Source: CAD feature listing. Evaluate the final solid. Frame: model axes, mm. A direction names the side the tool comes from. Round coordinates to 2 decimals unless told otherwise and drop trailing zeros. Loops run counter-clockwise (first coordinate to the right, second up) from the corner with the lowest first, then second, coordinate; pieces in that order, holes last.
Item 1: Section query B-B on z = 46.99. Return loops of the section in (x, y), then the cut area to 3 significant figures.
Item 2: Access query for faces 5 (the cylindrical face through (13.91, 0.8, -30.83)), 6 (the flat face through (0.783, 25.561, 17.647)), 7 (the cylindrical face through (1.36, 1.43, -3.94)). Directions: +Z, -Z, +X, -X, +Y, -Y. A direction counts if a zero-diameter tool reaches every point of the face in a straight line with its end or side. Return the directions, or none.
Item 3: Section query A-A on y = 12.7. Return loops of the section in (x, z), then the cut area to 3 significant figures.
Item 4: Ray query, L1, parallel to Y at x = 1, z = 14.5; L2, parallel to Y at x = 4.5, z = -15; L3, parallel to X at y = 97.5, z = 24. Return the intervals inside material, ascending.
Item 5: Section query D-D on x = 14. Return loops of the section in (y, z), then the cut area to 3 significant figures.
Item 6: Pull-direction query (Z, two-part tool) for faces 1 (the flat face through (20, 1.588, -4)), 2 (the flat face through (1, 61, -40.64)), 3 (the cylindrical face through (0.78, 105.47, 17.82)), 4 (the flat face through (0.783, 46.246, 17.647)); classes: released by +Z, released by -Z, zero draft, split by the parting line, or undercut.
Item 7: First-contact query: P1, Ø1.7, axis at x = 0.5, y = 102, coming from the +Z side; P2, Ø1.5, axis at x = 15, z = -25, coming from the +Y side; P3, Ø2, axis at x = 3, z = 13.5, coming from the +Y side. Flat tips, straight axial feed; report the tip coordinate or a pass-through.
```python
from build123d import *

# Parameters (mm, degrees)
SKETCH2_R                     = 14.2875
SKETCH2_R_2                   = 2.54
BOSS_EXTRUDE1_DEPTH           = 1.5875
SKETCH7_W                     = 1.5875
SKETCH7_H                     = 27.94
CUT_EXTRUDE1_DEPTH            = 0.00254
EDGE_FLANGE2_STRIP_W          = 12.7
EDGE_FLANGE2_STRIP_H          = 1.5875
EDGE_FLANGE2_STRIP_CUT_DEPTH  = 72.39
EDGE_FLANGE2_RELIEF_W         = 13.49375
EDGE_FLANGE2_RELIEF_H         = 0.79375
EDGE_FLANGE2_RELIEF_CUT_DEPTH = 1.5875
EDGE_FLANGE2_DEPTH            = 72.39
SKETCH14_R                    = 2.54
CUT_EXTRUDE2_DEPTH            = 2.54


# Sheet-metal steps are written as plain solids
with BuildPart() as part:
    # Sketch2 → Boss-Extrude1 (new body)
    with BuildSketch(Plane(origin=(0, 0, 0), x_dir=(0, 0, -1), z_dir=(1, 0, 0))):
        Polygon((-59.69, 95.25), (-59.69, 0), (40.64, 0), (40.64, 95.25), (40.64, 120.65), (-31.75, 120.65), (-31.75, 95.25), align=None)
        with Locations((0, 80.264)):
            Circle(SKETCH2_R, mode=Mode.SUBTRACT)
        with Locations((-46.99, 80.264)):
            Circle(SKETCH2_R_2, mode=Mode.SUBTRACT)
        with Locations((-46.99, 63.373)):
            Circle(SKETCH2_R_2, mode=Mode.SUBTRACT)
        with Locations((-17.272, 107.95)):
            Circle(SKETCH2_R_2, mode=Mode.SUBTRACT)
        with Locations((-2.794, 107.95)):
            Circle(SKETCH2_R_2, mode=Mode.SUBTRACT)
        with Locations((11.684, 107.95)):
            Circle(SKETCH2_R_2, mode=Mode.SUBTRACT)
        with Locations((26.162, 107.95)):
            Circle(SKETCH2_R_2, mode=Mode.SUBTRACT)
        with Locations((-46.99, 46.482)):
            Circle(SKETCH2_R_2, mode=Mode.SUBTRACT)
        with Locations((-46.99, 29.591)):
            Circle(SKETCH2_R_2, mode=Mode.SUBTRACT)
        with Locations((-46.99, 12.7)):
            Circle(SKETCH2_R_2, mode=Mode.SUBTRACT)
        with BuildLine():
            Line((-27.305, 64.866068321), (-8.255, 53.867545693))
            ThreePointArc((-8.255, 53.867545693), (-7.62, 52.76769343), (-8.255, 51.667841167))
            Line((-8.255, 51.667841167), (-27.305, 40.669318539))
            ThreePointArc((-27.305, 40.669318539), (-28.575, 40.669318539), (-29.21, 41.769170802))
            Line((-29.21, 41.769170802), (-29.21, 63.766216058))
            ThreePointArc((-29.21, 63.766216058), (-28.575, 64.866068321), (-27.305, 64.866068321))
        make_face(mode=Mode.SUBTRACT)
        with BuildLine():
            Line((-6.35, 43.235640486), (-6.35, 21.238595229))
            ThreePointArc((-6.35, 21.238595229), (-6.985, 20.138742967), (-8.255, 20.138742967))
            Line((-8.255, 20.138742967), (-27.305, 31.137265595))
            ThreePointArc((-27.305, 31.137265595), (-27.94, 32.237117857), (-27.305, 33.33697012))
            Line((-27.305, 33.33697012), (-8.255, 44.335492748))
            ThreePointArc((-8.255, 44.335492748), (-6.985, 44.335492748), (-6.35, 43.235640486))
        make_face(mode=Mode.SUBTRACT)
        with BuildLine():
            Line((8.255, 20.138742967), (27.305, 31.137265595))
            ThreePointArc((27.305, 31.137265595), (27.94, 32.237117857), (27.305, 33.33697012))
            Line((27.305, 33.33697012), (8.255, 44.335492748))
            ThreePointArc((8.255, 44.335492748), (6.985, 44.335492748), (6.35, 43.235640486))
            Line((6.35, 43.235640486), (6.35, 21.238595229))
            ThreePointArc((6.35, 21.238595229), (6.985, 20.138742967), (8.255, 20.138742967))
        make_face(mode=Mode.SUBTRACT)
        with BuildLine():
            Line((8.255, 51.667841167), (27.305, 40.669318539))
            ThreePointArc((27.305, 40.669318539), (28.575, 40.669318539), (29.21, 41.769170802))
            Line((29.21, 41.769170802), (29.21, 63.766216058))
            ThreePointArc((29.21, 63.766216058), (28.575, 64.866068321), (27.305, 64.866068321))
            Line((27.305, 64.866068321), (8.255, 53.867545693))
            ThreePointArc((8.255, 53.867545693), (7.62, 52.76769343), (8.255, 51.667841167))
        make_face(mode=Mode.SUBTRACT)
    extrude(amount=BOSS_EXTRUDE1_DEPTH)

    # Sketch7 → Cut-Extrude1 (cut)
    with BuildSketch(Plane(origin=(0, 0, 0), x_dir=(-1, 0, 0), z_dir=(0, -1, 0))):
        with Locations((-0.79375, -45.72)):
            Rectangle(SKETCH7_W, SKETCH7_H)
    extrude(amount=-CUT_EXTRUDE1_DEPTH, mode=Mode.SUBTRACT)

    # Edge-Flange2 strip (across the edge) → Edge-Flange2 strip cut (cut)
    with BuildSketch(Plane(origin=(1.5875, 0, 31.75), x_dir=(0, 1, 0), z_dir=(0, 0, -1))):
        with Locations((-1.5875, -0.79375)):
            Rectangle(EDGE_FLANGE2_STRIP_W, EDGE_FLANGE2_STRIP_H)
    extrude(amount=EDGE_FLANGE2_STRIP_CUT_DEPTH, mode=Mode.SUBTRACT)

    # Edge-Flange2 relief (on the sheet) → Edge-Flange2 relief cut (cut)
    with BuildSketch(Plane(origin=(1.5875, 4.7625, 31.75), x_dir=(0, 1, 0), z_dir=(1, 0, 0))):
        with Locations((-5.953125, 0.396875)):
            Rectangle(EDGE_FLANGE2_RELIEF_W, EDGE_FLANGE2_RELIEF_H)
    extrude(amount=-EDGE_FLANGE2_RELIEF_CUT_DEPTH, mode=Mode.SUBTRACT)

    # Edge-Flange2 section (across the edge) → Edge-Flange2 (add)
    with BuildSketch(Plane(origin=(1.5875, 0, 31.75), x_dir=(0, 1, 0), z_dir=(0, 0, -1))):
        with BuildLine():
            Line((0, 3.175), (0, 23.8125))
            Line((0, 23.8125), (1.5875, 23.8125))
            Line((1.5875, 23.8125), (1.5875, 3.175))
            ThreePointArc((1.5875, 3.175), (2.51743597, 0.92993597), (4.7625, 0))
            Line((4.7625, 0), (4.7625, -1.5875))
            ThreePointArc((4.7625, -1.5875), (1.394903955, -0.192596045), (0, 3.175))
        make_face()
    extrude(amount=EDGE_FLANGE2_DEPTH)

    # Sketch14 → Cut-Extrude2 (cut)
    with BuildSketch(Plane(origin=(0, 1.5875, 0), x_dir=(1, 0, 0), z_dir=(0, 1, 0))):
        with Locations(Location((15.08125, -19.685, 0), (0, 0, 180))):
            Circle(SKETCH14_R)
        with Locations(Location((15.08125, -7.62, 0), (0, 0, 180))):
            Circle(SKETCH14_R)
        with Locations(Location((15.08125, 4.445, 0), (0, 0, 180))):
            Circle(SKETCH14_R)
        with Locations(Location((15.08125, 16.51, 0), (0, 0, 180))):
            Circle(SKETCH14_R)
        with Locations(Location((15.08125, 28.575, 0), (0, 0, 180))):
            Circle(SKETCH14_R)
    extrude(amount=-CUT_EXTRUDE2_DEPTH, mode=Mode.SUBTRACT)


solid = part.part
```
Data:
1. outline: (0, 0) - (1.59, 0) - (1.59, 10.16) - (0, 10.16) - close; (0, 15.24) - (1.59, 15.24) - (1.59, 27.05) - (0, 27.05) - close; (0, 32.13) - (1.59, 32.13) - (1.59, 43.94) - (0, 43.94) - close; (0, 49.02) - (1.59, 49.02) - (1.59, 60.83) - (0, 60.83) - close; (0, 65.91) - (1.59, 65.91) - (1.59, 77.72) - (0, 77.72) - close; (0, 82.8) - (1.59, 82.8) - (1.59, 95.25) - (0, 95.25) - close
1. area: 111 mm2
2. face 5: +Y, -Y
2. face 6: +X, -X
2. face 7: -Z, -X, -Y
3. outline: (0, -40.64) - (1.59, -40.64) - (1.59, 44.45) - (0, 44.45) - close; (0, 49.53) - (1.59, 49.53) - (1.59, 59.69) - (0, 59.69) - close
3. area: 151 mm2
4. L1: y = 1.84 to 23.74, 40.73 to 48.06, 57.47 to 120.65
4. L2: y = 0.01 to 1.6
4. L3: x = 0 to 1.59
5. outline: (0, -40.64) - (1.59, -40.64) - (1.59, -30.87) - (0, -30.87) - close; (0, -26.28) - (1.59, -26.28) - (1.59, -18.81) - (0, -18.81) - close; (0, -14.21) - (1.59, -14.21) - (1.59, -6.74) - (0, -6.74) - close; (0, -2.15) - (1.59, -2.15) - (1.59, 5.32) - (0, 5.32) - close; (0, 9.92) - (1.59, 9.92) - (1.59, 17.39) - (0, 17.39) - close; (0, 21.98) - (1.59, 21.98) - (1.59, 31.75) - (0, 31.75) - close
5. area: 78.4 mm2
6. face 1: zero draft
6. face 2: released by -Z
6. face 3: undercut
6. face 4: undercut
7. P1: stops at z = 31.75
7. P2: stops at y = 1.59
7. P3: stops at y = 3.2
